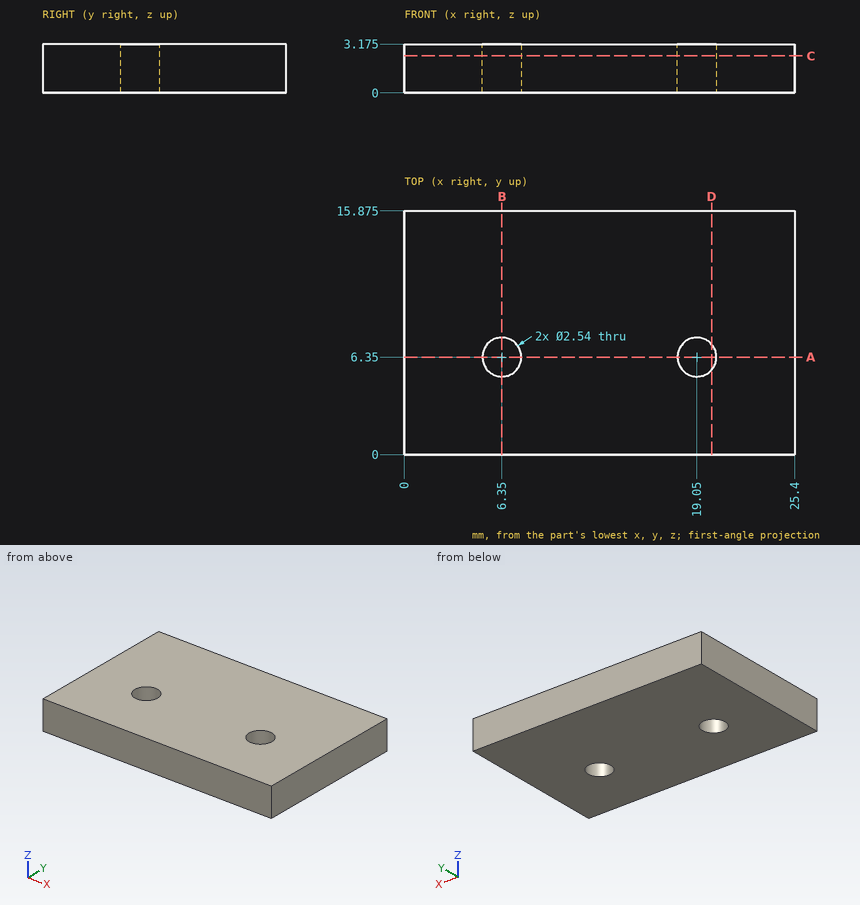
Check sheet for the drawn part. Datum: minimum x, y, z corner. Units: mm. Give positions to 0.01 mm unless a question says otherwise; leave off trailing zeros. Write each loop counter-clockwise with the first axis right and the second up, starting at its lowest first coordinate (ties: lowest second). Pieces come first, ordered by that corner, then holes.
(1) Cross-section at A-A (y = 6.35). Enter the section's corners in (x, z) (3 decimals).
(2) Cross-section at C-C (z = 2.4). Enter the section's corners in (x, y) (3 decimals), plus the area to 3 significant figures.
(3) Cross-section at B-B (x = 6.35). Enter the section's corners in (y, z) (3 decimals), plus the area to 3 significant figures.
(4) Material ranges on line 1 (Y direction, x = 19.05, z = 0.9) (3 decimals); line 2 (Y direction, x = 5.25, z = 2.6) (3 decimals), recorded low to high.
(5) Cross-section at D-D (x = 20). Enter the section's corners in (y, z) (3 decimals).
Worked out:
1. outline: (0, 0) - (5.08, 0) - (5.08, 3.175) - (0, 3.175) - close; (7.62, 0) - (17.78, 0) - (17.78, 3.175) - (7.62, 3.175) - close; (20.32, 0) - (25.4, 0) - (25.4, 3.175) - (20.32, 3.175) - close
2. outline: (0, 0) - (25.4, 0) - (25.4, 15.875) - (0, 15.875) - close; hole circle Ø2.54 at (6.35, 6.35); hole circle Ø2.54 at (19.05, 6.35)
2. area: 393 mm2
3. outline: (0, 0) - (5.08, 0) - (5.08, 3.175) - (0, 3.175) - close; (7.62, 0) - (15.875, 0) - (15.875, 3.175) - (7.62, 3.175) - close
3. area: 42.3 mm2
4. line 1: y = 0 to 5.08, 7.62 to 15.875
4. line 2: y = 0 to 5.715, 6.985 to 15.875
5. outline: (0, 0) - (5.507, 0) - (5.507, 3.175) - (0, 3.175) - close; (7.193, 0) - (15.875, 0) - (15.875, 3.175) - (7.193, 3.175) - close
